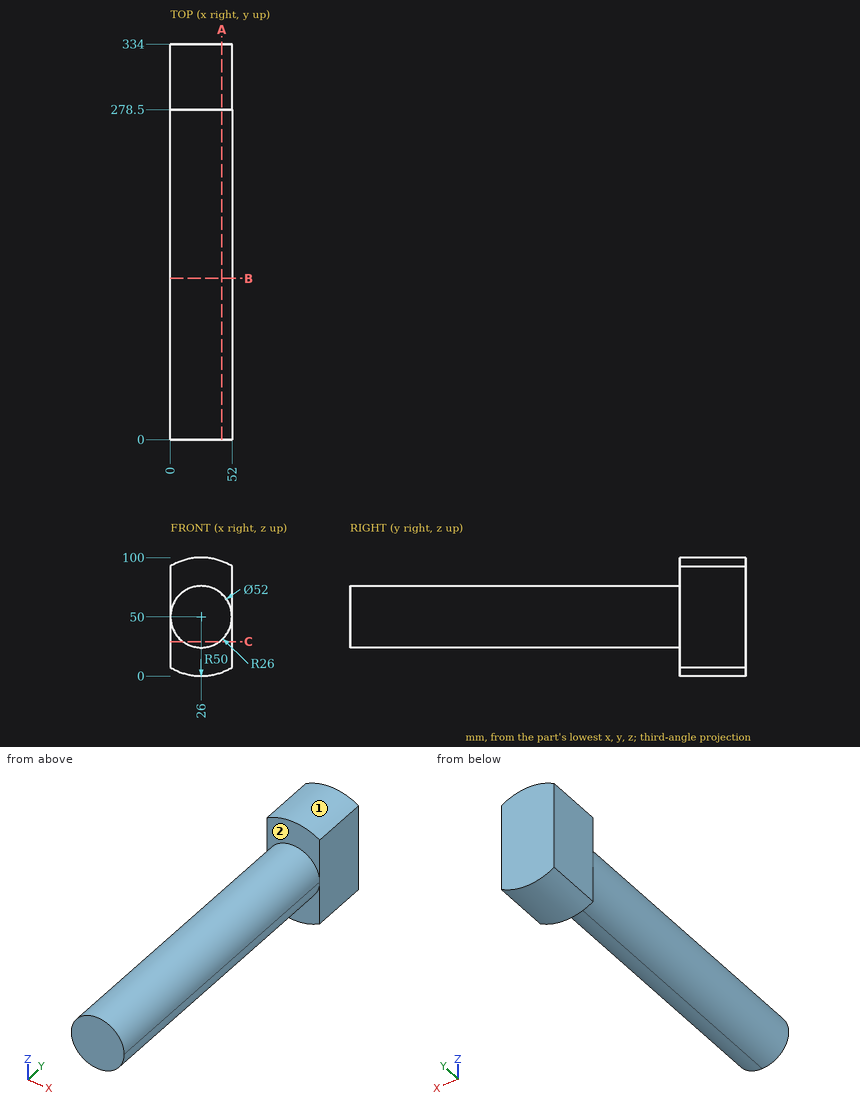
Print and shaded views of the part. All mm, measured from the part's lowest x, y and z. A direction names the side the tool comes from. Coordinates: 2 decimals unless noted, no trailing zeros. Order: outer loops, then holes, each group sorted by start corner. A loop starts at its lowest first (then second) coordinate and runs counter-clockwise, first axis right, second up. Notation, with made-up numbers: M 38.25,72.5 L 77.25,72.5 A22 cw 77.25,85.5 Z; hole C -31,-24.75 d7. An arc over 180 degrees is marked long. One line per question, with ' | ' between items. Start each with the question number.
Q1. 3-axis set-ups, long thin cutter, end or side, ignore diameter. For the marked faces 1 and 2: which of +Z, -Z, +X, -X, +Y, -Y reach the whole face in a straight line?
Q2. Probe L1, parallel to Y at x = 26.5, z = 16; L2, parallel to Z at x = 26.5, y = 135; L3, parallel to Z at x = 34, y = 218. List the from-to ranges inside material, lowest first. Write a range as from..to.
Q3. Flat gauge pins, fed straight in: pin 1 Ø1.5 at (x, y) = (6, 262) entering from -Z; pin 2 Ø1 at (x, y) = (8, 152.5) entering from +Z; pin 3 Ø2 at (x, y) = (9.5, 229.5) entering from -Z. Where does each tip first touch, or does it go through?
Q4. Saw through at C-C (z = 29). List the corners of the cut face in (x, y), then the cut area to 3 significant figures.
Q5. Saw through at B-B (y = 136). List the corners of the cut face in (x, z).
Q6. Saw through at A-A (x = 43.5). List the corners of the cut face in (y, z), then the cut area to 3 significant figures.
Check values:
1) face 1: +Z, +Y, -Y | face 2: +Z, -Y
2) L1: y = 278.5..334 | L2: z = 24..76 | L3: z = 25.26..74.74
3) pin 1: stops at z = 32.52 | pin 2: stops at z = 69.23 | pin 3: stops at z = 29.13
4) outline: M 0,278.5 L 10.67,278.5 L 10.67,0 L 41.33,0 L 41.33,278.5 L 52,278.5 L 52,334 L 0,334 Z | area: 11,400 mm2
5) outline: C 26,50 d52
6) outline: M 0,30.77 L 278.5,30.77 L 278.5,3.16 L 334,3.16 L 334,96.84 L 278.5,96.84 L 278.5,69.23 L 0,69.23 Z | area: 15,900 mm2
